Model file for the job. Use its own axes, mm. Coordinates: 2 decimals unless noted, no trailing zeros. Loops run counter-clockwise (first coordinate to the right, second up) from the corner with the lowest first, then second, coordinate; pieces in that order, holes last.
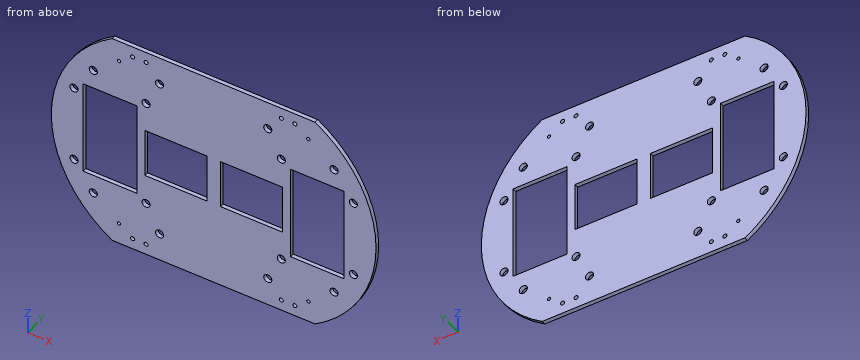
Autodesk Inventor part; units mm, degrees
ref_plane "YZ Plane" through (0, 0, 0) normal (1, 0, 0) x (0, 1, 0)
ref_plane "XZ Plane" through (0, 0, 0) normal (0, 1, 0) x (-1, 0, 0)
ref_plane "XY Plane" through (0, 0, 0) normal (0, 0, 1) x (1, 0, 0)
sketch "Esquisse1" plane through (0, 0, 0) normal (0, 1, 0) x (-1, 0, 0)
  circle A0 centre (0, 0) radius 25 construction
  line L0 (-25, 0) -> (25, 0) construction
  arc A1 (-75, -80.7775) -> (-75, 80.7775) centre (-25, 0) ccw construction
  arc A2 (75, 80.7775) -> (75, -80.7775) centre (25, 0) ccw construction
  line L1 (0, 25) -> (0, 0) construction
  line L2 (-75, 80.7775) -> (75, 80.7775)
  line L3 (-75, -80.7775) -> (75, -80.7775)
  arc A3 (75, -80.7775) -> (75, 80.7775) centre (25, 0) ccw
  arc A4 (-75, 80.7775) -> (-75, -80.7775) centre (-25, 0) ccw
  dimension "d0" = 50
  dimension "d1" = 190
  dimension "d2" = 150
extrude "Extrusion1" add sketch "Esquisse1" along normal blind 3
sketch "Esquisse4" plane through (0, 0, 0) normal (0, -1, 0) x (1, 0, 0)
  line L0 (-50, 40) -> (50, 40) construction
  line L1 (50, 40) -> (50, -40) construction
  line L2 (50, -40) -> (-50, -40) construction
  line L3 (-50, -40) -> (-50, 40) construction
  circle A0 centre (-50, 40) radius 3
  circle A1 centre (50, 40) radius 3
  circle A2 centre (50, -40) radius 3
  circle A3 centre (-50, -40) radius 3
  line L4 (75, 80.7775) -> (-75, 80.7775)
  point P0 (0, 0)
  dimension "d15" = 80
  dimension "d16" = 100
  dimension "d17" = 50
  dimension "d18" = 40
  dimension "d19" = 6
  dimension "d20" = 6
  dimension "d21" = 6
  dimension "d22" = 6
  dimension "d25" = 40.7775
extrude "Extrusion4" cut sketch "Esquisse4" against normal through all
sketch "Esquisse5" plane through (0, 0, 0) normal (0, -1, 0) x (1, 0, 0)
  arc A0 (-75, 80.7775) -> (-75, -80.7775) centre (-25, 0) ccw
  line L0 (-96.5, 35) -> (-70.8, 35)
  line L1 (-70.8, 35) -> (-70.8, -35)
  line L2 (-70.8, -35) -> (-96.5, -35)
  line L3 (-96.5, -35) -> (-96.5, 35)
  line L4 (-70.8, 35) -> (-66.8, 35)
  line L5 (-66.8, 35) -> (-66.8, -35)
  line L6 (-66.8, -35) -> (-70.8, -35)
  line L7 (-70.8, -35) -> (-70.8, 35)
  line L8 (-66.8, 35) -> (-56.8, 35)
  line L9 (-56.8, 35) -> (-56.8, -35)
  line L10 (-56.8, -35) -> (-66.8, -35)
  line L11 (-66.8, -35) -> (-66.8, 35)
  line L12 (0, 0) -> (-120, 0) construction
  dimension "d26" = 4
  dimension "d27" = 70
  dimension "d28" = 35
  dimension "d29" = 25.7
  dimension "d30" = 10
  dimension "d31" = 23.5
  dimension "d80" = 56.8
extrude "Extrusion5" cut sketch "Esquisse5" against normal through all
mirror "Symétrie1" about plane through (0, 0, 0) normal (1, 0, 0) of "Extrusion5"
sketch "Esquisse8" plane through (0, 0, 0) normal (0, -1, 0) x (1, 0, 0)
  line L0 (96.5, 35) -> (96.5, -35)
  line L1 (82, 42) -> (96, 42)
  line L2 (96, 42) -> (96, -42)
  line L3 (96, -42) -> (82, -42)
  line L4 (82, -42) -> (82, 42)
  line L5 (96, 21.5) -> (108.5, 21.5)
  line L6 (108.5, 21.5) -> (108.5, -21.5)
  line L7 (108.5, -21.5) -> (96, -21.5)
  line L8 (96, -21.5) -> (96, 21.5)
  line L9 (82, -14.7) -> (76.3, -14.7)
  line L10 (76.3, -14.7) -> (76.3, 14.7)
  line L11 (76.3, 14.7) -> (82, 14.7)
  line L12 (82, 14.7) -> (82, -14.7)
  line L13 (82, 14.7) -> (72, 14.7)
  line L14 (72, 14.7) -> (72, 24.7)
  line L15 (72, 24.7) -> (82, 24.7)
  line L16 (82, 24.7) -> (82, 14.7)
  line L17 (96, 21.5) -> (110.5, 21.5)
  line L18 (110.5, 21.5) -> (110.5, 35.5)
  line L19 (110.5, 35.5) -> (96, 35.5)
  line L20 (96, 35.5) -> (96, 21.5)
  line L21 (96, 42) -> (82, 42)
  line L22 (82, 42) -> (82, 56)
  line L23 (82, 56) -> (96, 56)
  line L24 (96, 56) -> (96, 42)
  line L25 (72, 24.7) -> (82, 14.7) construction
  line L26 (82, 24.7) -> (72, 14.7) construction
  line L27 (110.5, 21.5) -> (96, 35.5) construction
  line L28 (96, 21.5) -> (110.5, 35.5) construction
  line L29 (82, 56) -> (96, 42) construction
  line L30 (82, 42) -> (96, 56) construction
  circle A0 centre (89, 49) radius 3
  circle A1 centre (77, 19.7) radius 3
  circle A2 centre (103.25, 28.5) radius 3
  arc A3 (75, -80.7775) -> (75, 80.7775) centre (25, 0) ccw
  line L31 (108.5, 21.5) -> (115, 21.5)
  line L32 (115, 21.5) -> (115, -21.5)
  line L33 (115, -21.5) -> (108.5, -21.5)
  line L34 (108.5, -21.5) -> (108.5, 21.5)
  line L35 (0, 0) -> (120, 0)
  dimension "d59" = 84
  dimension "d60" = 14
  dimension "d61" = 29.4
  dimension "d62" = 5.7
  dimension "d63" = 12.5
  dimension "d64" = 43
  dimension "d65" = 42
  dimension "d66" = 14.7
  dimension "d67" = 21.5
  dimension "d68" = 14
  dimension "d69" = 14
  dimension "d70" = 14
  dimension "d71" = 10
  dimension "d72" = 10
  dimension "d73" = 6
  dimension "d74" = 6
  dimension "d75" = 6
  dimension "d78" = 6.5
  dimension "d79" = 5
extrude "Extrusion6" cut sketch "Esquisse8" against normal through all contours A0 | A1 | A2
mirror "Symétrie2" about plane through (0, 0, 0) normal (0, 0, 1) of "Extrusion6"
mirror "Symétrie3" about plane through (0, 0, 0) normal (1, 0, 0) of "Extrusion6", "Symétrie2"
sketch "Esquisse9" plane through (0, 0, 0) normal (0, -1, 0) x (1, 0, 0)
  line L0 (56.8, -35) -> (56.8, 35)
  line L1 (5, 18) -> (50.8, 18)
  line L2 (50.8, 18) -> (50.8, -18)
  line L3 (50.8, -18) -> (5, -18)
  line L4 (5, -18) -> (5, 18)
  point P0 (0, 0)
  dimension "d81" = 36
  dimension "d82" = 18
  dimension "d83" = 6
  dimension "d84" = 5
extrude "Extrusion7" cut sketch "Esquisse9" against normal through all
mirror "Symétrie4" about plane through (0, 0, 0) normal (1, 0, 0) of "Extrusion7"
sketch "Esquisse10" plane through (0, 0, 0) normal (0, -1, 0) x (1, 0, 0)
  circle A0 centre (70, 65) radius 1.25
  point P0 (0, 0)
  dimension "d87" = 65
  dimension "d88" = 70
  dimension "d89" = 2.5
extrude "Extrusion8" cut sketch "Esquisse10" against normal through all
mirror "Symétrie5" about plane through (0, 0, 0) normal (1, 0, 0) of "Extrusion8"
mirror "Symétrie6" about plane through (0, 0, 0) normal (0, 0, 1) of "Extrusion8", "Symétrie5"
sketch "Esquisse11" plane through (0, 0, 0) normal (0, -1, 0) x (1, 0, 0)
  line L0 (-65, 79.7775) -> (-45, 79.7775)
  line L1 (-45, 79.7775) -> (-45, 69.7775)
  line L2 (-45, 69.7775) -> (-65, 69.7775)
  line L3 (-65, 69.7775) -> (-65, 79.7775)
  line L4 (-75, 80.7775) -> (75, 80.7775)
  circle A0 centre (-70, 65) radius 1.25
  circle A1 centre (-70, 65) radius 10
  circle A2 centre (-60, 72.7775) radius 1.5
  circle A3 centre (-50, 72.7775) radius 1.5
  point P0 (0, 0)
  dimension "d92" = 10
  dimension "d93" = 20
  dimension "d94" = 1
  dimension "d95" = 5
  dimension "d96" = 20
  dimension "d97" = 3
  dimension "d98" = 3
  dimension "d99" = 3
  dimension "d100" = 3
  dimension "d101" = 5
  dimension "d102" = 5
extrude "Extrusion9" cut sketch "Esquisse11" against normal through all contours A2 | A3
mirror "Symétrie7" about plane through (0, 0, 0) normal (1, 0, 0) of "Extrusion9"
mirror "Symétrie8" about plane through (0, 0, 0) normal (0, 0, 1) of "Extrusion9", "Symétrie7"
sketch "Esquisse12" plane through (0, 0, 0) normal (0, -1, 0) x (1, 0, 0)
  line L0 (-40, 60) -> (40, 60) construction
  line L1 (40, 60) -> (40, -60) construction
  line L2 (40, -60) -> (-40, -60) construction
  line L3 (-40, -60) -> (-40, 60) construction
  circle A0 centre (-40, 60) radius 3
  circle A1 centre (40, 60) radius 3
  circle A2 centre (-40, -60) radius 3
  circle A3 centre (40, -60) radius 3
  point P0 (0, 0)
  dimension "d105" = 80
  dimension "d106" = 120
  dimension "d107" = 60
  dimension "d108" = 40
  dimension "d109" = 6
  dimension "d110" = 6
  dimension "d111" = 6
  dimension "d112" = 6
extrude "Extrusion10" cut sketch "Esquisse12" against normal through all
equation "\"d20\" = d19"
equation "\"d21\" = d19"
equation "\"d22\" = d19"
equation "\"d28\" = 0.5 * d27"
equation "\"d65\" = 0.5 * d59"
equation "\"d66\" = 0.5 * d61"
equation "\"d67\" = 0.5 * d64"
equation "\"d68\" = d60"
equation "\"d70\" = d69"
properties part number "base"
Q1. Slice it at C-C (x = -40). List the corners of the cut face in (y, z).
Answers:
outline: (0, -80.78) - (3, -80.78) - (3, -63) - (0, -63) - close; (0, -57) - (3, -57) - (3, -18) - (0, -18) - close; (0, 18) - (3, 18) - (3, 57) - (0, 57) - close; (0, 63) - (3, 63) - (3, 80.78) - (0, 80.78) - close
Q2. Slice it at A-A (z = 0). List the corners of the cut face in (x, y).
Answers:
outline: (-120, 0) - (-96.5, 0) - (-96.5, 3) - (-120, 3) - close; (-56.8, 0) - (-50.8, 0) - (-50.8, 3) - (-56.8, 3) - close; (-5, 0) - (5, 0) - (5, 3) - (-5, 3) - close; (50.8, 0) - (56.8, 0) - (56.8, 3) - (50.8, 3) - close; (96.5, 0) - (120, 0) - (120, 3) - (96.5, 3) - close
Q3. Slice it at B-B (x = 28). List the corners of the cut face in (y, z).
Answers:
outline: (0, -80.78) - (3, -80.78) - (3, -18) - (0, -18) - close; (0, 18) - (3, 18) - (3, 80.78) - (0, 80.78) - close
Q4. Flat gauge pins, fed straight in: P1, Ø9.5, axis at x = -103.25, z = 28.5, coming from the -Y side; P2, Ø0.9, axis at y = 2, z = 3.5, coming from the -X side; P3, Ø1.5, axis at x = -85.5, y = 1, coming from the +Z side; P4, Ø2.5, axis at x = 50, z = 72.78, coming from the +Y side. Where does each tip first touch, or does it go through?
Answers:
P1: stops at y = 0
P2: stops at x = -119.95
P3: stops at z = 73.86
P4: passes through
Q5. Slice it at D-D (z = -49). List the corners of the cut face in (x, y), and give its area (3 significant figures).
Answers:
outline: (-106.39, 0) - (-92, 0) - (-92, 3) - (-106.39, 3) - close; (-86, 0) - (86, 0) - (86, 3) - (-86, 3) - close; (92, 0) - (106.39, 0) - (106.39, 3) - (92, 3) - close
area: 602 mm2
Q6. Drill centre lines: line 1 (Z direction, x = 50, y = 1.35); line 2 (Z direction, x = -40, y = 2.15); line 3 (Z direction, x = -66.5, y = 0.25). Where is each one in solid material? Low to high.
Answers:
line 1: z = -80.78 to -74.28, -71.28 to -43, -37 to -18, 18 to 37, 43 to 71.28, 74.28 to 80.78
line 2: z = -80.78 to -63, -57 to -18, 18 to 57, 63 to 80.78
line 3: z = -80.78 to -35, 35 to 80.78
